```python
from build123d import *

# Parameters (mm, degrees)
F1_DEPTH = 8
F6_W     = 6.3
F6_H     = 3.3
F7_DEPTH = 11.9
F8_DEPTH = 7


with BuildPart() as f1:
    # F0 (on Top) → F1 (new body)
    with BuildSketch(Plane.XY):
        with BuildLine():
            Line((9.259995, 5.75), (8.785642, 5.75))
            Line((8.785642, 5.75), (-8.785642, 5.75))
            Line((-8.785642, 5.75), (-9.259995, 5.75))
            ThreePointArc((-9.259995, 5.75), (-10.9, 0), (-9.259995, -5.75))
            Line((-9.259995, -5.75), (-8.785642, -5.75))
            Line((-8.785642, -5.75), (8.785642, -5.75))
            Line((8.785642, -5.75), (9.259995, -5.75))
            ThreePointArc((9.259995, -5.75), (10.9, 0), (9.259995, 5.75))
        make_face()
    extrude(amount=-F1_DEPTH)

    # F2 (on face) → F5 section 0
    with BuildSketch(Plane.XZ.offset(5.75)):
        Polygon((1.9, 0), (-1.9, 0), (-2.9, -2), (2.9, -2), align=None)
    # F4 (on offset) → F5 section 1
    with BuildSketch(Plane.XZ.offset(-3)):
        Polygon((2.5, -2), (1.5, 0), (-1.5, 0), (-2.5, -2), align=None)
    loft(mode=Mode.SUBTRACT)

    # F6 (on Right) → F7 (cut)
    with BuildSketch(Plane.YZ):
        with Locations((0, -5.15)):
            Rectangle(F6_W, F6_H)
    extrude(amount=-F7_DEPTH, mode=Mode.SUBTRACT)

    # F6 (on Right) → F8 (cut)
    with BuildSketch(Plane.YZ):
        with Locations((0, -5.15)):
            Rectangle(F6_W, F6_H)
    extrude(amount=F8_DEPTH, mode=Mode.SUBTRACT)


solid = f1.part
```
Geometry check sheet. Reference: the model listing, model coordinates, mm. A direction names the side the tool comes from. Coordinates: 2 decimals unless noted, no trailing zeros. Write each loop counter-clockwise with the first axis right and the second up, starting at its lowest first coordinate (ties: lowest second). Pieces come first, ordered by that corner, then holes. Notation, with made-up numbers: M 20,79.25 L 25,79.25 A20 cw 25,99.25 Z; hole C 28,-12.75 d11. An arc over 180 degrees is marked long. Answer as a JSON object with one key per item and string values.
1. Tool access check on faces 5 (the flat face through (0, 3, -1)), 6 (the flat face through (-2, -3.15, -5)), 7 (the cylindrical face through (10.9, -0.1, -3.9)). Record the directions out of +Z, -Z, +X, -X, +Y, -Y that give a thin tool (end or side, any length) a straight path to the whole face; none if there is none.
Answers below:
{"face 5": "-Y", "face 6": "-X", "face 7": "+Z, -Z, +X"}
2. Go/stop test with flat-tipped pins: pin 1 Ø4 at (y, z) = (3, -2) entering from -X; pin 2 Ø1.6 at (y, z) = (1, -5.5) entering from -X; pin 3 Ø3 at (y, z) = (4, -5) entering from +X. Record where each tip stops, or that it passes through.
Answers below:
{"pin 1": "stops at x = -10.85", "pin 2": "stops at x = 7", "pin 3": "stops at x = 10.61"}
3. Draft check along Z on faces 1 (the flat face through (0, 0, -8)), 2 (the flat face through (2, 0, 0)), 3 (the flat face through (7, 0, -5)), 4 (the flat face through (0, 5.75, -4)). Enter one of: released by +Z, released by -Z, zero draft, split by the parting line, or undercut.
Answers below:
{"face 1": "released by -Z", "face 2": "released by +Z", "face 3": "undercut", "face 4": "zero draft"}
4. Scan lines: L1, parallel to Z at x = -1, y = -2.5; L2, parallel to Z at x = -9.75, y = 3; L3, parallel to Y at x = -9, z = -4.5. Record each from-to range of solid material in increasing order.
Answers below:
{"L1": "z = -8 to -6.8, -3.5 to -2", "L2": "z = -8 to -6.8, -3.5 to 0", "L3": "y = -5.75 to -3.15, 3.15 to 5.75"}
5. Section check B-B, the plane z = -5. Enter the section's corners in (x, y), plus the area to 3 significant figures.
Answers below:
{"outline": "M -10.43,-3.15 A10.9 ccw -9.26,-5.75 L 9.26,-5.75 A10.9 ccw 9.26,5.75 L -9.26,5.75 A10.9 ccw -10.43,3.15 L 7,3.15 L 7,-3.15 Z", "area": "127 mm²"}
6. Section check A-A, the plane x = -5.5. Enter the section's corners in (y, z), plus the area to 3 significant figures.
Answers below:
{"outline": "M -5.75,-8 L 5.75,-8 L 5.75,0 L -5.75,0 Z; hole M -3.15,-6.8 L 3.15,-6.8 L 3.15,-3.5 L -3.15,-3.5 Z", "area": "71.2 mm²"}
